Read the model definition and answer for the solid it produces. Units are mm, in the model's axes. A direction names the side the tool comes from. Coordinates: 2 decimals unless noted, no trailing zeros. Answer as a JSON object with one key per item and string values. Group by question number.
1) Determine the mould class of faces 1 (the face through (214.6, 36, 10)), 2 (the face through (224.6, 25, 0)), 3 (the face through (219.67, 39.766, -9.879)) for opening direction Z: released by +Z, released by -Z, zero draft, split by the parting line, or undercut.
2) Flat-ended cylindrical pins translate along their axes: P1, Ø2.5, axis at y = 36, z = -10.5, coming from the -X side; P2, Ø5, axis at y = 35.8, z = 10.4, coming from the +X side. Find the tip coordinate at first contact, or state that the pin passes through.
3) Consider probe 1 along Y at (x, z) = (222, 10.4); probe 2 along Z at (x, y) = (-222, 35); probe 3 along X at (y, z) = (18, -8). Determine where each line is inside the solid, lowest interval first. Write a range as [from, to].
4) Which of the six approach directions +Z, -Z, +X, -X, +Y, -Y give full straight-line access (tool end or side, diameter ignored) to faces 4 (the face through (-3, 50.8, 0)), 5 (the face through (219.67, 39.766, 10.921)), 6 (the face through (-214.6, 36, -10))?
from build123d import *

# Parameters (mm, degrees)
CROQUIS1_W              = 449.2
CROQUIS1_H              = 50.8
SALIENTE_EXTRUIR1_DEPTH = 50.8
CROQUIS2_R              = 4
CORTAR_EXTRUIR1_DEPTH   = 10
CROQUIS3_R              = 4
CORTAR_EXTRUIR2_DEPTH   = 10


with BuildPart() as part:
    # Croquis1 → Saliente-Extruir1 (new body)
    with BuildSketch(Plane(origin=(0, 0, 0), x_dir=(1, 0, 0), z_dir=(0, 1, 0))):
        Rectangle(CROQUIS1_W, CROQUIS1_H)
    extrude(amount=SALIENTE_EXTRUIR1_DEPTH)

    # Croquis2 → Cortar-Extruir1 (cut)
    with BuildSketch(Plane(origin=(224.6, 0, 0), x_dir=(0, 0, -1), z_dir=(1, 0, 0))):
        with Locations((-10.4, 35.8)):
            Circle(CROQUIS2_R)
        with Locations((10.4, 35.8)):
            Circle(CROQUIS2_R)
        with Locations((10.4, 15)):
            Circle(CROQUIS2_R)
        with Locations((-10.4, 15)):
            Circle(CROQUIS2_R)
    extrude(amount=-CORTAR_EXTRUIR1_DEPTH, mode=Mode.SUBTRACT)

    # Croquis3 → Cortar-Extruir2 (cut)
    with BuildSketch(Plane.ZY.offset(224.6)):
        with Locations((10.4, 35.8)):
            Circle(CROQUIS3_R)
        with Locations((-10.4, 35.8)):
            Circle(CROQUIS3_R)
        with Locations((-10.4, 15)):
            Circle(CROQUIS3_R)
        with Locations((10.4, 15)):
            Circle(CROQUIS3_R)
    extrude(amount=-CORTAR_EXTRUIR2_DEPTH, mode=Mode.SUBTRACT)


solid = part.part
Determined:
{
 "1": {"face 1": "undercut", "face 2": "zero draft", "face 3": "undercut"},
 "2": {"P1": "x = -214.6", "P2": "x = 214.6"},
 "3": {"probe 1": "[0, 11], [19, 31.8], [39.8, 50.8]", "probe 2": "[-25.4, -14.32], [-6.48, 6.48], [14.32, 25.4]", "probe 3": "[-214.6, 214.6]"},
 "4": {"face 4": "+Z, -Z, +X, -X, +Y", "face 5": "+X", "face 6": "-X"}
}
